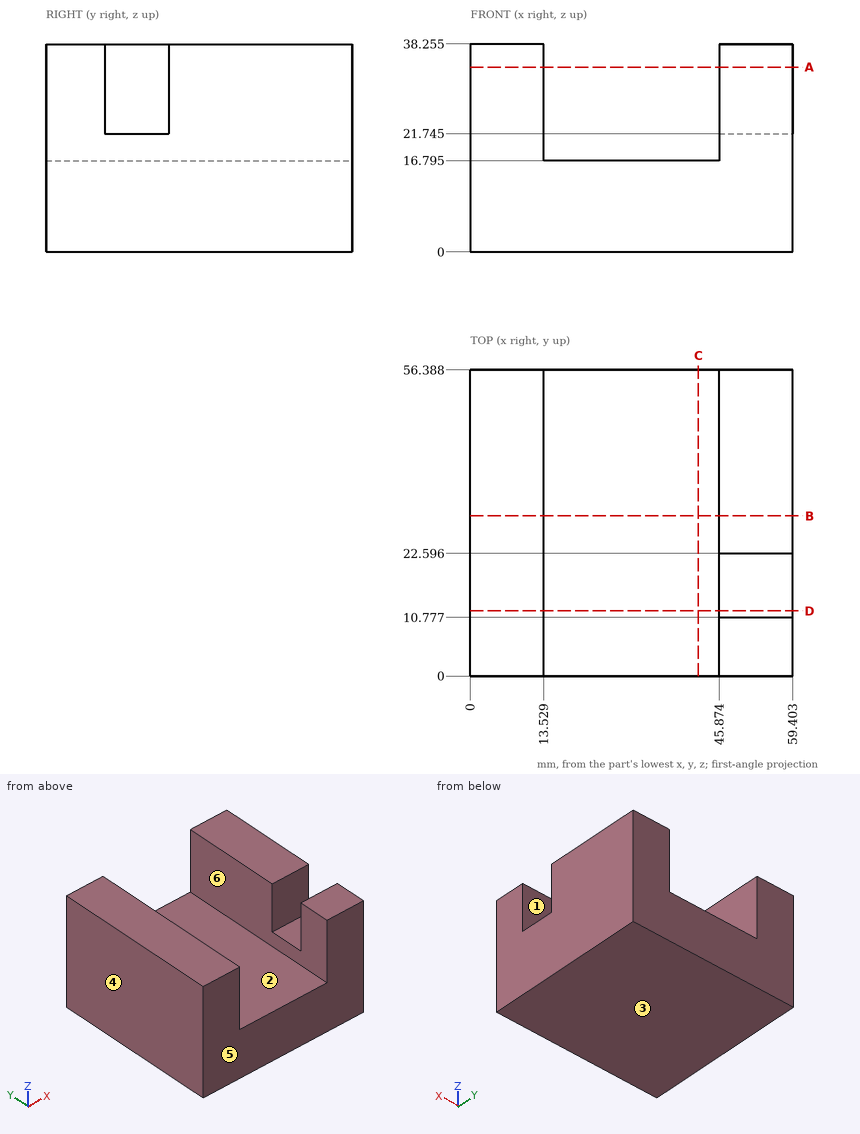
Could you check a few things on this drawing? It's one solid part, dimensions in mm from its lowest x, y, z. A direction names the side the tool comes from. Coordinates: 2 decimals unless noted, no trailing zeros. Loops run counter-clockwise (first coordinate to the right, second up) from the corner with the lowest first, then second, coordinate; pieces in that order, holes last. Notation, with made-up numbers: (-27.5, 55.25) - (-6.5, 55.25) arc R24 cw to (-6.5, 84.25) - close; hole circle Ø3 at (-21, 48). An arc over 180 degrees is marked (long way). Answer as a JSON object with one key per item and string values. Group by question number.
Item 1: For pin 1 (1.5 mm diameter, centred on x = 15.5, z = 18.5, fed in from -Y); pin 2 (9.5 mm diameter, centred on x = 25.5, y = 22, fed in from +Z) (1 decimal); pin 3 (6 mm diameter, centred on x = 55.5, y = 17, fed in from +Z) (1 decimal), each with a flat end and sliding along its axis, tell me the tip position at first contact or that it passes through.
Item 2: If we section it at A-A (z = 34): List the corners of the cut face in (x, y) for me (1 decimal).
Item 3: If we section it at B-B (y = 29.5): List the corners of the cut face in (x, z) for me (1 decimal).
Item 4: If we section it at C-C (x = 42): List the corners of the cut face in (y, z) for me (1 decimal).
Item 5: On a 3-axis mill with a long thin cutter (end or side, diameter ignored), from which of +Z, -Z, +X, -X, +Y, -Y can I reach the whole of each face in a straight line? I mean the marked faces 1, 2 and 3. Say none if no direction works.
Item 6: If we mould it in two halves opening along X, with no side actions, what happens to the marked faces 4, 5 and 6? For each: released by +X, released by -X, zero draft, split by the parting line, or undercut.
Item 7: If we section it at D-D (y = 12): List the corners of the cut face in (x, z) for me (1 decimal).
Item 8: If I drill on L1, parallel to X at y = 29, z = 29.5 (1 decimal); L2, parallel to Z at x = 14.5, y = 21 (1 decimal), over which ranges is the centre line in solid material (lowest first)? Write a range as from..to.
Returned:
{
 "1": {"pin 1": "passes through", "pin 2": "stops at z = 16.8", "pin 3": "stops at z = 21.7"},
 "2": {"outline": "(0, 0) - (13.5, 0) - (13.5, 56.4) - (0, 56.4) - close; (45.9, 0) - (59.4, 0) - (59.4, 10.8) - (45.9, 10.8) - close; (45.9, 22.6) - (59.4, 22.6) - (59.4, 56.4) - (45.9, 56.4) - close"},
 "3": {"outline": "(0, 0) - (59.4, 0) - (59.4, 38.3) - (45.9, 38.3) - (45.9, 16.8) - (13.5, 16.8) - (13.5, 38.3) - (0, 38.3) - close"},
 "4": {"outline": "(0, 0) - (56.4, 0) - (56.4, 16.8) - (0, 16.8) - close"},
 "5": {"face 1": "+Z, +X", "face 2": "+Z, +Y, -Y", "face 3": "-Z, +X, -X, +Y, -Y"},
 "6": {"face 4": "released by -X", "face 5": "zero draft", "face 6": "undercut"},
 "7": {"outline": "(0, 0) - (59.4, 0) - (59.4, 21.7) - (45.9, 21.7) - (45.9, 16.8) - (13.5, 16.8) - (13.5, 38.3) - (0, 38.3) - close"},
 "8": {"L1": "x = 0..13.5, 45.9..59.4", "L2": "z = 0..16.8"}
}
